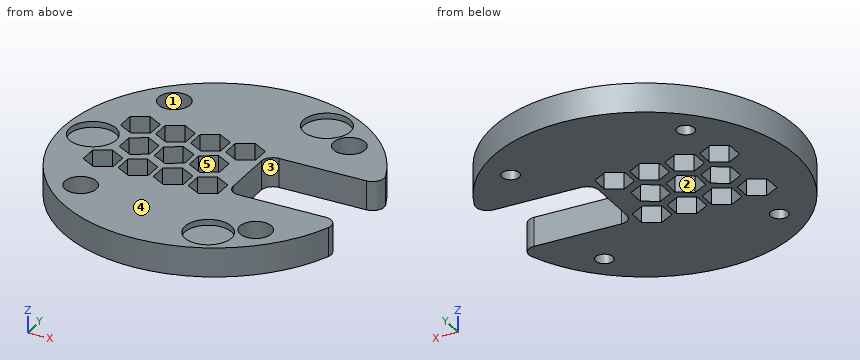
from build123d import *

# Parameters (mm, degrees)
SKETCH_R        = 25.999973
PAD_DEPTH       = 5
SKETCH001_R     = 1.5
POCKET_DEPTH    = 5.001
SKETCH002_W     = 20.5
SKETCH002_H     = 13.007144
POCKET001_DEPTH = 5
FILLET_R        = 2
POCKET002_DEPTH = 5
SKETCH004_R     = 4.000249
SKETCH004_R_2   = 4
POCKET003_DEPTH = 1
SKETCH005_R     = 2.7
POCKET004_DEPTH = 3


with BuildPart() as part:
    # Sketch → Pad (new body)
    with BuildSketch(Plane.XY):
        Circle(SKETCH_R)
    extrude(amount=PAD_DEPTH)

    # Sketch001 (on Face3 of Pad) → Pocket (cut, through all)
    with BuildSketch(Plane.XY.offset(5)):
        with Locations((-15, 15)):
            Circle(SKETCH001_R)
        with Locations((15, 15)):
            Circle(SKETCH001_R)
        with Locations((15, -15)):
            Circle(SKETCH001_R)
        with Locations((-15, -15)):
            Circle(SKETCH001_R)
    extrude(amount=-POCKET_DEPTH, mode=Mode.SUBTRACT)

    # Sketch002 (on Face3 of Pocket) → Pocket001 (cut)
    with BuildSketch(Plane.XY.offset(5)):
        with Locations((15.75, 0.027864)):
            Rectangle(SKETCH002_W, SKETCH002_H)
    extrude(amount=-POCKET001_DEPTH, mode=Mode.SUBTRACT)

    # Fillet
    fillet_edges = [part.edges().sort_by_distance(p)[0] for p in [
        (5.5, 6.531436, 2.5),
        (5.5, -6.475708, 2.5),
        (25.180624, -6.475708, 2.5),
        (25.166226, 6.531436, 2.5),
    ]]
    fillet(fillet_edges, radius=FILLET_R)

    # Sketch003 (on Face5 of Fillet) → Pocket002 (cut)
    with BuildSketch(Plane.XY.offset(5)):
        Polygon((-16, 9), (-18.598076, 7.5), (-18.598076, 4.5), (-16, 3), (-13.401924, 4.5), (-13.401924, 7.5), align=None)
        Polygon((-10, 9), (-12.598076, 7.5), (-12.598076, 4.5), (-10, 3), (-7.401924, 4.5), (-7.401924, 7.5), align=None)
        Polygon((-4, 9), (-6.598076, 7.5), (-6.598076, 4.5), (-4, 3), (-1.401924, 4.5), (-1.401924, 7.5), align=None)
        Polygon((2, 9), (-0.598076, 7.5), (-0.598076, 4.5), (2, 3), (4.598076, 4.5), (4.598076, 7.5), align=None)
        Polygon((-12.990973, 3), (-15.593563, 1.507818), (-15.60259, -1.492182), (-13.009027, -3), (-10.406437, -1.507818), (-10.39741, 1.492182), align=None)
        Polygon((-7.054188, 3), (-9.62517, 1.453072), (-9.570982, -1.546928), (-6.945812, -3), (-4.37483, -1.453072), (-4.429018, 1.546928), align=None)
        Polygon((-1.012141, 3), (-3.604147, 1.489486), (-3.592006, -1.510514), (-0.987859, -3), (1.604147, -1.489486), (1.592006, 1.510514), align=None)
        Polygon((-16, -3), (-18.598076, -4.5), (-18.598076, -7.5), (-16, -9), (-13.401924, -7.5), (-13.401924, -4.5), align=None)
        Polygon((-10, -3), (-12.598076, -4.5), (-12.598076, -7.5), (-10, -9), (-7.401924, -7.5), (-7.401924, -4.5), align=None)
        Polygon((-4, -3), (-6.598076, -4.5), (-6.598076, -7.5), (-4, -9), (-1.401924, -7.5), (-1.401924, -4.5), align=None)
        Polygon((2, -3), (-0.598076, -4.5), (-0.598076, -7.5), (2, -9), (4.598076, -7.5), (4.598076, -4.5), align=None)
    extrude(amount=-POCKET002_DEPTH, mode=Mode.SUBTRACT)

    # Sketch004 (on Face5 of Pocket002) → Pocket003 (cut)
    with BuildSketch(Plane.XY.offset(5)):
        with Locations((-20.955366, 0)):
            Circle(SKETCH004_R)
        with Locations((9, 19)):
            Circle(SKETCH004_R_2)
        with Locations((9, -19)):
            Circle(SKETCH004_R_2)
    extrude(amount=-POCKET003_DEPTH, mode=Mode.SUBTRACT)

    # Sketch005 (on Face5 of Pocket003) → Pocket004 (cut)
    with BuildSketch(Plane.XY.offset(5)):
        with Locations((-15, 15)):
            Circle(SKETCH005_R)
        with Locations((15, 15)):
            Circle(SKETCH005_R)
        with Locations((15, -15)):
            Circle(SKETCH005_R)
        with Locations((-15, -15)):
            Circle(SKETCH005_R)
    extrude(amount=-POCKET004_DEPTH, mode=Mode.SUBTRACT)


solid = part.part
The listing builds one solid part. Answer for the finished solid, in the listing's coordinates (mm). Face numbers are marked on the shaded views. A direction names the side the tool comes from. Coordinates: 2 decimals unless noted, no trailing zeros. Write each loop counter-clockwise with the first axis right and the second up, starting at its lowest first coordinate (ties: lowest second). Pieces come first, ordered by that corner, then holes. Notation, with made-up numbers: M 15.5,-6.75 L 58.5,-6.75 A32 ccw 58.5,24.25 Z; hole C -20.75,-4 d8. An arc over 180 degrees is marked long. Put each result on its own line as item: value. Start each with the question number.
1. Flat-ended cylindrical pins translate along their axes: P1, Ø2.5, axis at x = 15.5, y = -14, coming from the +Z side; P2, Ø1.5, axis at y = -5.5, z = 2, coming from the +X side; P3, Ø2, axis at y = 14, z = 3.5, coming from the -X side. Find the tip coordinate at first contact, or state that the pin passes through.
2. Consider line 1 (Y direction, x = 9, z = 4.05); line 2 (X direction, y = -5.5, z = 2.75); line 3 (X direction, y = -4.5, z = 2.3). Determine where each line is inside the solid, lowest interval first. Write a range as from..to.
3. A cutting plane is placed at A-A on y = 0. Write down the section's boundary in (x, z), then the cut area to 3 significant figures.
4. For a pull along Y with two mould halves and no side action, classify the marked faces 4 and 5 as pulls with the +Y half, pulls with the -Y half, needs draft (parallel to the pull), parting line crosses it, or undercut.
5. A cutting plane is placed at B-B on x = -15. Count the separate pieces of the cut face and the enclosed holes in it, then the cut area to 3 significant figures.
6. A cutting plane is placed at C-C on x = 9. Write down the section's boundary in (y, z), then the cut area to 3 significant figures.
7. Which of the six approach directions +Z, -Z, +X, -X, +Y, -Y give full straight-line access (tool end or side, diameter ignored) to the marked faces 1, 2 and 3?
8. A cutting plane is placed at D-D on x = 15. Write down the section's boundary in (y, z).
Resolved:
1. P1: stops at z = 2
1. P2: stops at x = 6.58
1. P3: stops at x = -22.52
2. line 1: y = -24.39..-23, -15..-6.48, 6.53..15, 23..24.39
2. line 2: x = -25.41..-18.6, -13.4..-12.6, -7.4..-6.6, -1.4..-0.6, 4.6..5.78
2. line 3: x = -25.61..-18.6, -13.4..-12.6, -7.4..-6.6, -1.4..-0.6, 4.6..5.5
3. outline: M -26,0 L -15.6,0 L -15.6,5 L -16.96,5 L -16.96,4 L -24.96,4 L -24.96,5 L -26,5 Z; M -10.4,0 L -9.6,0 L -9.6,5 L -10.4,5 Z; M -4.4,0 L -3.6,0 L -3.6,5 L -4.4,5 Z; M 1.6,0 L 5.5,0 L 5.5,5 L 1.6,5 Z
3. area: 71.5 mm2
4. face 4: needs draft
4. face 5: undercut
5. separate pieces: 6
5. enclosed holes: 0
5. area: 101 mm2
6. outline: M -24.39,0 L -6.48,0 L -6.48,5 L -15,5 L -15,4 L -23,4 L -23,5 L -24.39,5 Z; M 6.53,0 L 24.39,0 L 24.39,5 L 23,5 L 23,4 L 15,4 L 15,5 L 6.53,5 Z
6. area: 163 mm2
7. face 1: +Z
7. face 2: +Z, -Z
7. face 3: +Z, -Z, +X
8. outline: M -21.24,0 L -16.5,0 L -16.5,2 L -17.7,2 L -17.7,5 L -21.24,5 Z; M -13.5,0 L -6.48,0 L -6.48,5 L -12.3,5 L -12.3,2 L -13.5,2 Z; M 6.53,0 L 13.5,0 L 13.5,2 L 12.3,2 L 12.3,5 L 6.53,5 Z; M 16.5,0 L 21.24,0 L 21.24,5 L 17.7,5 L 17.7,2 L 16.5,2 Z
